from build123d import *

# Parameters (mm, degrees)
F1_ANGLE      = 30
F2_R          = 3.81
F3_DEPTH      = 100.331
F3_DEPTH_BACK = 100.331
F4_W          = 5.08
F4_H          = 15.24
F5_DEPTH      = 2.54


with BuildPart() as f1:
    # F0 (on Top) → F1 (revolve)
    with BuildSketch(Plane.XY):
        with BuildLine():
            Line((-100.33, 0), (-95.25, 0))
            ThreePointArc((-95.25, 0), (0, 95.25), (95.25, 0))
            Line((95.25, 0), (100.33, 0))
            ThreePointArc((100.33, 0), (0, 100.33), (-100.33, 0))
        make_face()
    revolve(axis=Axis((-47.625, 0, 0), (1, 0, 0)), revolution_arc=F1_ANGLE)

    # F2 (on Right) → F3 (cut, two sides)
    with BuildSketch(Plane.YZ) as f3_sk:
        Circle(F2_R)
    extrude(amount=-F3_DEPTH, mode=Mode.SUBTRACT)
    extrude(f3_sk.sketch, amount=F3_DEPTH_BACK, mode=Mode.SUBTRACT)

    # F4 (on Top) → F5 (join)
    with BuildSketch(Plane.XY):
        with Locations((-0.3907692308, 95.2049005657)):
            Rectangle(F4_W, F4_H)
    extrude(amount=F5_DEPTH)


solid = f1.part
Design review of the part built by this model. Coordinates are the model's own, in mm. Round coordinates to 2 decimals unless told otherwise and drop trailing zeros. Write each loop counter-clockwise with the first axis right and the second up, starting at its lowest first coordinate (ties: lowest second). Pieces come first, ordered by that corner, then holes. Notation, with made-up numbers: M 29,47.25 L 71,47.25 A18 cw 71,64.25 Z; hole C 2,81 d8. An arc over 180 degrees is marked long. One line per item, written item: value. Start each with the question number.
1. Take a section at A-A on y = 21. State the section outline as (x, z) points, then the cut area to 3 significant figures.
2. Take a section at C-C on z = 42.5. State the section outline as (x, y) points.
3. To check wall thickness, follow probe 1 along X at (y, z) = (65.5, 23); probe 2 along X at (y, z) = (78.5, 34); probe 3 along Y at (x, z) = (57, 33). State the ranges of each line that lie inside material, in increasing order. Write a range as from..to.
4. Take a section at D-D on x = 57. State the section outline as (y, z) points.
5. Take a section at B-B on y = 82. State the section outline as (x, z) points, then the cut area to 3 significant figures.
6. Clearance check with flat-ended pins moving along their axes: P1, Ø2, axis at x = 34.5, z = 30, coming from the +Y side; P2, Ø12, axis at x = -34.5, z = 6, coming from the -Y side; P3, Ø1, axis at x = 23, y = 87.5, coming from the +Z side; P4, Ø2, axis at x = 66, y = 79, coming from the +Z side. State where each tip first meets the part, or that it passes through.
7. Draft analysis for pull direction Z (two halves, no side actions). For faces 1 (the face through (0, 90, 0)), 2 (the face through (0, 91, 2.54)), 3 (the face through (-7.894, 82.44, 47.596)), state which applies: pulls with the +Z half, pulls with the -Z half, needs draft (parallel to the pull), parting line crosses it, or undercut.
Computed:
1. outline: M -98.11,0 L -92.91,0 A92.91 cw -92.11,12.12 L -97.36,12.12 A98.11 ccw Z; M 92.11,12.12 A92.91 cw 92.91,0 L 98.11,0 A98.11 ccw 97.36,12.12 Z
1. area: 126 mm²
2. outline: M -53.3,73.61 L -42.98,73.61 A85.24 cw 42.98,73.61 L 53.3,73.61 A90.88 ccw Z
3. probe 1: x = -72.44..-65.22, 65.22..72.44
3. probe 2: x = -52.42..-41.88, 41.88..52.42
3. probe 3: y = 68.81..75.68
4. outline: M 66.09,38.16 A76.31 cw 76.31,0 L 82.57,0 A82.57 ccw 71.5,41.28 Z
5. outline: M -57.81,0 L -48.46,0 A48.46 cw -10.36,47.34 L -33.18,47.34 A57.81 ccw Z; M 10.36,47.34 A48.46 cw 48.46,0 L 57.81,0 A57.81 ccw 33.18,47.34 Z
5. area: 1,100 mm²
6. P1: stops at y = 89.81
6. P2: stops at y = 85.97
6. P3: stops at z = 44.4
6. P4: passes through
7. face 1: pulls with the -Z half
7. face 2: undercut
7. face 3: pulls with the +Z half
